Part model, mm, in its own coordinate system. A direction names the side the tool comes from. Coordinates: 2 decimals unless noted, no trailing zeros. Order: outer loops, then holes, each group sorted by start corner. A loop starts at its lowest first (then second) coordinate and runs counter-clockwise, first axis right, second up.
1) Mould opens along X. For faces 4 (the flat face through (-29, 63, -6)), 5 (the cylindrical face through (-23.862, 57.217, -7.521)), 6 (the cylindrical face through (-27.142, 62.725, -13.733)), 7 (the cylindrical face through (-27.87, 63.29, -7.52)) say: +X half, -X half, draft (parallel to the pull), parting line (faces both ways), or undercut.
2) Wall check: L1, parallel to Y at x = -27.5, z = -7.25; L2, parallel to Y at x = -27.5, z = -6.25; L3, parallel to Z at x = -31.5, y = 62.5. Give the ranges that are in metal, low to high.
3) Cut at C-C (z = -2). List the corners of the cut face in (x, y).
4) Cut at B-B (z = -8). List the corners of the cut face in (x, y).
5) Tool access for faces 1 (the flat face through (-29, 63, -9)), 2 (the cylindrical face through (-27.858, 62.725, -3.161)), 3 (the cylindrical face through (-26.2, 54.14, -7.48)): list every direction of +Z, -Z, +X, -X, +Y, -Y with a clear straight run to the whole face (end or side of a thin tool).
6) Pin check, flat tips, straight feed: pin 1 Ø1.3 at (x, y) = (-30.96, 58) entering from +Z; pin 2 Ø2 at (x, y) = (-27.5, 64) entering from -Z; pin 3 Ø4 at (x, y) = (-23, 57.5) entering from +Z. Stop position of each tip, or through.
7) Cut at A-A (x = -27.5). List the corners of the cut face in (y, z), and give its area (3 significant figures).
```python
from build123d import *

# Parameters (mm, degrees)
SKETCH1_R             = 2.75
BOSS_EXTRUDE1_DEPTH   = 6
SKETCH3_R             = 6
BOSS_EXTRUDE2_DEPTH   = 3
SKETCH4_R             = 2.75
BOSS_EXTRUDE3_DEPTH   = 10
M2X0_4_TAPPED_HOLE1_D = 1.6
CHAMFER1_SIZE         = 0.4
SKETCH7_R             = 2
CUT_EXTRUDE1_DEPTH    = 20


with BuildPart() as part:
    # Sketch1 → Boss-Extrude1 (new body)
    with BuildSketch(Plane.XY):
        with Locations((-27.5, 59.99791663)):
            Circle(SKETCH1_R)
    extrude(amount=-BOSS_EXTRUDE1_DEPTH)

    # Sketch3 → Boss-Extrude2 (add)
    with BuildSketch(Plane(origin=(0, 0, -6), x_dir=(-1, 0, 0), z_dir=(0, 0, -1))):
        with Locations((27.5, 59.99791663)):
            Circle(SKETCH3_R)
    extrude(amount=BOSS_EXTRUDE2_DEPTH)

    # Sketch4 → Boss-Extrude3 (add)
    with BuildSketch(Plane(origin=(0, 0, -9), x_dir=(-1, 0, 0), z_dir=(0, 0, -1))):
        with Locations((27.5, 59.99791663)):
            Circle(SKETCH4_R)
    extrude(amount=BOSS_EXTRUDE3_DEPTH)

    # M2x0.4 Tapped Hole1 (through all)
    with Locations(Plane.XY.offset(-6)):
        with Locations((-24.035898385, 57.99791663), (-30.964101615, 57.99791663), (-27.5, 63.99791663)):
            Hole(M2X0_4_TAPPED_HOLE1_D / 2)

    # Chamfer1
    chamfer1_edges = [part.edges().sort_by_distance(p)[0] for p in [
        (-24.75, 59.99791663, -19),
        (-30.25, 59.99791663, 0),
        (-21.5, 59.99791663, -6),
        (-21.5, 59.99791663, -9),
    ]]
    chamfer(chamfer1_edges, length=CHAMFER1_SIZE)

    # Sketch7 → Cut-Extrude1 (cut, through all)
    with BuildSketch(Plane.XY):
        with Locations((-27.5, 59.99791663)):
            Circle(SKETCH7_R)
    extrude(amount=-CUT_EXTRUDE1_DEPTH, mode=Mode.SUBTRACT)


solid = part.part
```
Geometry check:
1. face 4: draft
1. face 5: undercut
1. face 6: parting line
1. face 7: undercut
2. L1: y = 54 to 58, 62 to 63.2, 64.8 to 66
2. L2: y = 54.15 to 58, 62 to 63.2, 64.8 to 65.85
2. L3: z = -9 to -6
3. outline: circle Ø5.5 at (-27.5, 60); hole circle Ø4 at (-27.5, 60)
4. outline: circle Ø12 at (-27.5, 60); hole circle Ø1.6 at (-30.96, 58); hole circle Ø4 at (-27.5, 60); hole circle Ø1.6 at (-27.5, 64); hole circle Ø1.6 at (-24.04, 58)
5. face 1: -Z
5. face 2: +Z
5. face 3: +Z, -Z
6. pin 1: passes through
6. pin 2: stops at z = -9
6. pin 3: stops at z = -6
7. outline: (54, -8.6) - (54.4, -9) - (57.25, -9) - (57.25, -18.6) - (57.65, -19) - (58, -19) - (58, 0) - (57.65, 0) - (57.25, -0.4) - (57.25, -6) - (54.4, -6) - (54, -6.4) - close; (62, -19) - (62.35, -19) - (62.75, -18.6) - (62.75, -9) - (63.2, -9) - (63.2, -6) - (62.75, -6) - (62.75, -0.4) - (62.35, 0) - (62, 0) - close; (64.8, -9) - (65.6, -9) - (66, -8.6) - (66, -6.4) - (65.6, -6) - (64.8, -6) - close
7. area: 42.6 mm2
